Design review of the part built by this model. Coordinates are the model's own, in mm. Face numbers are marked on the shaded views. Give positions to 0.01 mm unless a question says otherwise; leave off trailing zeros. Loops run counter-clockwise (first coordinate to the right, second up) from the corner with the lowest first, then second, coordinate; pieces in that order, holes last. Notation, with made-up numbers: (86, 40.5) - (143, 40.5) arc R21 cw to (143, 59.5) - close; hole circle Ø4 at (82.25, 86). An arc over 180 degrees is marked (long way). One line per item, written item: value. Start each with the question number.
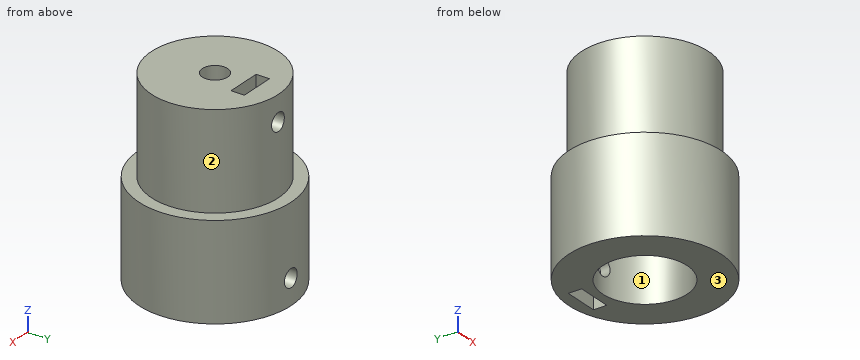
```python
from build123d import *

# Parameters (mm, degrees)
F0_R      = 12
F0_R_2    = 6.65
F1_DEPTH  = 15
F3_R      = 1.4
F4_DEPTH  = 10
F5_R      = 10
F5_R_2    = 2
F6_DEPTH  = 15
F8_R      = 1.4
F9_DEPTH  = 11
F10_W     = 5.5
F10_H     = 2.1
F11_DEPTH = 8.5
F12_W     = 5.5
F12_H     = 2.1
F13_DEPTH = 8.5


# Not quite as in the source:
# - a feature names something its author has since deleted; it is built from what else it names


with BuildPart() as f1:
    # F0 (on Top) → F1 (new body)
    with BuildSketch(Plane.XY):
        Circle(F0_R)
        Circle(F0_R_2, mode=Mode.SUBTRACT)
    extrude(amount=F1_DEPTH)

    # F3 (on offset) → F4 (cut)
    with BuildSketch(Plane.XZ.offset(-14)):
        with Locations((0, 4)):
            Circle(F3_R)
    extrude(amount=F4_DEPTH, mode=Mode.SUBTRACT)

    # F5 (on face) → F6 (join)
    with BuildSketch(Plane.XY.offset(15)):
        Circle(F5_R)
        Circle(F5_R_2, mode=Mode.SUBTRACT)
    extrude(amount=F6_DEPTH)

    # F8 (on offset) → F9 (cut)
    with BuildSketch(Plane.XZ.offset(-11.5)):
        with Locations((0, 26)):
            Circle(F8_R)
    extrude(amount=F9_DEPTH, mode=Mode.SUBTRACT)

    # F10 (on face) → F11 (cut)
    with BuildSketch(Plane.XY.offset(30)):
        with Locations((0, 5.55)):
            Rectangle(F10_W, F10_H)
    extrude(amount=-F11_DEPTH, mode=Mode.SUBTRACT)

    # F12 (on face) → F13 (cut)
    with BuildSketch(Plane.XY):
        with Locations((0, 9.05)):
            Rectangle(F12_W, F12_H)
    extrude(amount=F13_DEPTH, mode=Mode.SUBTRACT)


solid = f1.part
```
(1) Take a section at A-A on y = 0. State the section outline as (x, z) points.
(2) Take a section at C-C on y = 9. State the section outline as (x, z) points, and give its area (3 significant figures).
(3) To check wall thickness, follow L1, parallel to Z at x = 0, y = 7.6; L2, parallel to Z at x = 1, y = 6.75; L3, parallel to Z at x = 0, y = 10.9. State the ranges of each line that lie inside material, in increasing order. Write a range as from..to.
(4) For pin 1 Ø1.1 at (y, z) = (8.5, 3) entering from +X; pin 2 Ø3 at (x, y) = (0.5, 8) entering from -Z; pin 3 Ø2.5 at (x, z) = (0, 4) entering from +Y; pin 4 Ø6 at (y, z) = (-3.5, 7) entering from +X, all flat-tipped, find the tip position at first contact; note any pin that passes through.
(5) Draft analysis for pull direction X (two halves, no side actions). For the marked faces 1, 2 and 3, state which applies: pulls with the +X half, pulls with the -X half, needs draft (parallel to the pull), parting line crosses it, or undercut.
(6) Take a section at D-D on x = 7.25. State the section outline as (y, z) points, and give its area (3 significant figures).
(7) Take a section at B-B on z = 2. State the section outline as (x, y) points, and give its area (3 significant figures).
Here are the results:
1. outline: (-12, 0) - (-6.65, 0) - (-6.65, 15) - (-2, 15) - (-2, 30) - (-10, 30) - (-10, 15) - (-12, 15) - close; (2, 15) - (6.65, 15) - (6.65, 0) - (12, 0) - (12, 15) - (10, 15) - (10, 30) - (2, 30) - close
2. outline: (-7.94, 0) - (-2.75, 0) - (-2.75, 8.5) - (2.75, 8.5) - (2.75, 0) - (7.94, 0) - (7.94, 15) - (4.36, 15) - (4.36, 30) - (-4.36, 30) - (-4.36, 15) - (-7.94, 15) - close; hole circle Ø2.8 at (0, 26)
2. area: 316 mm²
3. L1: 0..2.6, 5.4..24.6, 27.4..30
3. L2: 0..3.02, 4.98..25.02, 26.98..30
3. L3: 0..2.6, 5.4..15
4. pin 1: x = 8.99
4. pin 2: z = 0
4. pin 3: y = -6.53
4. pin 4: x = 11.99
5. face 1: undercut
5. face 2: parting line crosses it
5. face 3: needs draft
6. outline: (-9.56, 0) - (9.56, 0) - (9.56, 15) - (6.89, 15) - (6.89, 30) - (-6.89, 30) - (-6.89, 15) - (-9.56, 15) - close
6. area: 493 mm²
7. outline: circle Ø24 at (0, 0); hole circle Ø13.3 at (0, 0); hole (-2.75, 8) - (2.75, 8) - (2.75, 10.1) - (-2.75, 10.1) - close
7. area: 302 mm²
